Geometry: final body of the model. Coordinates: model frame, mm. Face numbers are marked on the shaded views. A direction names the side the tool comes from. Coordinates: 2 decimals unless noted, no trailing zeros. Write each loop counter-clockwise with the first axis right and the second up, starting at its lowest first coordinate (ties: lowest second). Pieces come first, ordered by that corner, then holes. Notation, with made-up numbers: (-17, -22.5) - (-12, -22.5) arc R28 cw to (-12, -0.5) - close; hole circle Ø9 at (-36.75, 11.25). An arc over 180 degrees is marked (long way). Put each result on its own line as item: value.
```python
from build123d import *

# Parameters (mm, degrees)
PAD_DEPTH       = 3.175
SKETCH001_R     = 1.35
POCKET_DEPTH    = 3.176
POCKET001_DEPTH = 3.176


with BuildPart() as part:
    # Sketch → Pad (new body)
    with BuildSketch(Plane.XY):
        with BuildLine():
            ThreePointArc((-10.16, 8.89), (-11.956051, 8.146051), (-12.7, 6.35))
            Line((-12.7, -6.35), (-12.7, 6.35))
            ThreePointArc((-12.7, -6.35), (-11.956051, -8.146051), (-10.16, -8.89))
            Line((10.16, -8.89), (-10.16, -8.89))
            ThreePointArc((10.16, -8.89), (11.956051, -8.146051), (12.7, -6.35))
            Line((12.7, 6.35), (12.7, -6.35))
            ThreePointArc((12.7, 6.35), (11.956051, 8.146051), (10.16, 8.89))
            Line((-10.16, 8.89), (10.16, 8.89))
        make_face()
    extrude(amount=PAD_DEPTH)

    # Sketch001 → Pocket (cut, through all)
    with BuildSketch(Plane.XY):
        with Locations((-10.16, 6.35)):
            Circle(SKETCH001_R)
        with Locations((-10.16, -6.35)):
            Circle(SKETCH001_R)
        with Locations((10.16, 6.35)):
            Circle(SKETCH001_R)
        with Locations((10.16, -6.35)):
            Circle(SKETCH001_R)
    extrude(amount=POCKET_DEPTH, mode=Mode.SUBTRACT)

    # Sketch002 → Pocket001 (cut, through all)
    with BuildSketch(Plane.XY):
        Polygon((4.055886, -7.025), (8.111771, 0), (4.055886, 7.025), (-4.055886, 7.025), (-8.111771, 0), (-4.055886, -7.025), align=None)
    extrude(amount=POCKET001_DEPTH, mode=Mode.SUBTRACT)


solid = part.part
```
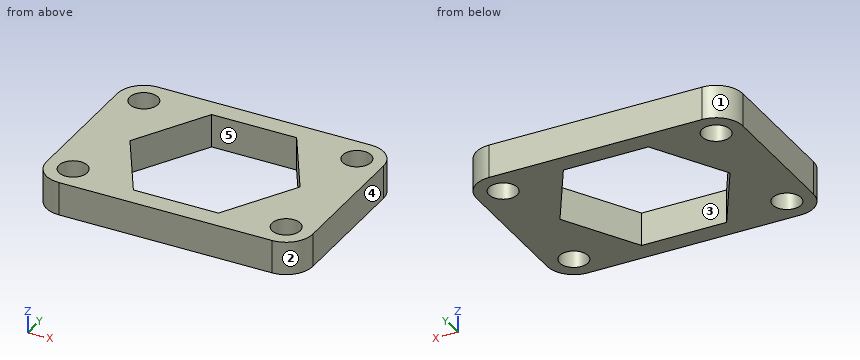
1. Section query A-A (x = 0.25). Return loops of the section in (y, z) (3 decimals).
Answer below:
outline: (-8.89, 0) - (-7.025, 0) - (-7.025, 3.175) - (-8.89, 3.175) - close; (7.025, 0) - (8.89, 0) - (8.89, 3.175) - (7.025, 3.175) - close
2. Ray query, probe 1 along Y at (x, z) = (-10.16, 0.85); probe 2 along Y at (x, z) = (9.25, 2.45); probe 3 along X at (y, z) = (6.35, 2.45). Return the intervals inside material, ascending. Write a range as from..to.
Answer below:
probe 1: y = -8.89..-7.7, -5..5, 7.7..8.89
probe 2: y = -8.89..-7.35, -5.35..5.35, 7.35..8.89
probe 3: x = -12.7..-11.51, -8.81..-4.45, 4.45..8.81, 11.51..12.7
3. Section query D-D (x = 11.25). Return loops of the section in (y, z) (1 decimal), then the cut area to 3 significant figures.
Answer below:
outline: (-8.6, 0) - (-7.1, 0) - (-7.1, 3.2) - (-8.6, 3.2) - close; (-5.6, 0) - (5.6, 0) - (5.6, 3.2) - (-5.6, 3.2) - close; (7.1, 0) - (8.6, 0) - (8.6, 3.2) - (7.1, 3.2) - close
area: 44.8 mm²
4. Mould query, pull axis X, two halves, no side actions, for the marked faces 1, 2 and 3. Classes: +X half, -X half, draft (parallel to the pull), parting line (faces both ways), or undercut.
Answer below:
face 1: -X half
face 2: +X half
face 3: undercut
5. Section query C-C (z = 2.3). Return loops of the section in (x, y) (3 decimals).
Answer below:
outline: (-12.7, -6.35) arc R2.54 ccw to (-10.16, -8.89) - (10.16, -8.89) arc R2.54 ccw to (12.7, -6.35) - (12.7, 6.35) arc R2.54 ccw to (10.16, 8.89) - (-10.16, 8.89) arc R2.54 ccw to (-12.7, 6.35) - close; hole circle Ø2.7 at (-10.16, -6.35); hole circle Ø2.7 at (-10.16, 6.35); hole (-8.112, 0) - (-4.056, -7.025) - (4.056, -7.025) - (8.112, 0) - (4.056, 7.025) - (-4.056, 7.025) - close; hole circle Ø2.7 at (10.16, -6.35); hole circle Ø2.7 at (10.16, 6.35)
6. Section query B-B (y = -2). Return loops of the section in (x, z) (3 decimals), then the cut area to 3 significant figures.
Answer below:
outline: (-12.7, 0) - (-6.957, 0) - (-6.957, 3.175) - (-12.7, 3.175) - close; (6.957, 0) - (12.7, 0) - (12.7, 3.175) - (6.957, 3.175) - close
area: 36.5 mm²
7. Set-up query: the marked faces 4 and 5. Return all of +Z, -Z, +X, -X, +Y, -Y with unobstructed straight access to the full face (end or side cutting, diameter ignored); none if empty.
Answer below:
face 4: +Z, -Z, +X, +Y, -Y
face 5: +Z, -Z
